Autodesk Inventor part; units mm, degrees
ref_plane "YZ Plane" through (0, 0, 0) normal (1, 0, 0) x (0, 1, 0)
ref_plane "XZ Plane" through (0, 0, 0) normal (0, 1, 0) x (-1, 0, 0)
ref_plane "XY Plane" through (0, 0, 0) normal (0, 0, 1) x (1, 0, 0)
sketch "Skizze1" plane through (0, 0, 0) normal (0, 0, 1) x (1, 0, 0)
  line L0 (-10.5, 14.5) -> (10.5, 14.5)
  line L1 (12.5, 12.5) -> (12.5, -7.362)
  line L2 (10.5, -9.362) -> (-10.5, -9.362)
  line L3 (-12.5, -7.362) -> (-12.5, 12.5)
  line L4 (-10.4, 12.5) -> (10.4, 12.5) construction
  line L5 (10.4, 12.5) -> (10.4, 0) construction
  line L6 (10.4, 0) -> (-10.4, 0) construction
  line L7 (-10.4, 0) -> (-10.4, 12.5) construction
  circle A0 centre (-10.4, 12.5) radius 1.1
  circle A1 centre (10.4, 12.5) radius 1.1
  circle A2 centre (-10.4, 0) radius 1.1
  circle A3 centre (10.4, 0) radius 1.1
  arc A4 (-10.5, 14.5) -> (-12.5, 12.5) centre (-10.5, 12.5) ccw
  arc A5 (12.5, 12.5) -> (10.5, 14.5) centre (10.5, 12.5) ccw
  arc A6 (10.5, -9.362) -> (12.5, -7.362) centre (10.5, -7.362) ccw
  arc A7 (-12.5, -7.362) -> (-10.5, -9.362) centre (-10.5, -7.362) ccw
  line L8 (0, -9.362) -> (0, 0) construction
  point P0 (-12.5, 14.5)
  point P1 (12.5, -9.362)
  point P2 (-12.5, -9.362)
  dimension "d0" = 25
  dimension "d1" = 23.862
  dimension "d2" = 2.2
  dimension "d3" = 2
  dimension "d4" = 20.8
  dimension "d5" = 12.5
  dimension "d6" = 2
extrude "Extrusion1" add sketch "Skizze1" along normal mid plane 1
sketch "Skizze2" plane through (0, 0, 0.5) normal (0, 0, 1) x (1, 0, 0)
  line L0 (-4.2, 4.2) -> (4.2, 4.2)
  line L1 (4.2, 4.2) -> (4.2, -4.2)
  line L2 (4.2, -4.2) -> (-4.2, -4.2)
  line L3 (-4.2, -4.2) -> (-4.2, 4.2)
  line L4 (-4.2, -4.2) -> (4.2, 4.2) construction
  point P0 (0, 0)
  point P1 (0, 0)
  dimension "d9" = 8.4
extrude "Extrusion2" add sketch "Skizze2" along normal blind 2.9
sketch "Skizze3" plane through (0, 0, 3.4) normal (0, 0, 1) x (1, 0, 0)
  circle A0 centre (0, 0) radius 3.6
  dimension "d12" = 7.2
extrude "Extrusion3" add sketch "Skizze3" along normal blind 1.7
sketch "Skizze4" plane through (0, 0, 5.1) normal (0, 0, 1) x (1, 0, 0)
  circle A0 centre (0, 0) radius 2.7
  circle A1 centre (0, 0) radius 0.85
  dimension "d15" = 5.4
  dimension "d16" = 1.7
extrude "Extrusion4" add sketch "Skizze4" along normal blind 0.5
sketch "Skizze5" plane through (0, 0, 0.5) normal (0, 0, 1) x (1, 0, 0)
  point P0 (0, 0)
sketch "Skizze6" plane through (0, 0, 0.5) normal (0, 0, 1) x (1, 0, 0)
  line L0 (4.2, 4.2) -> (-4.2, 4.2)
  line L1 (-3.5, 4.2) -> (3.5, 4.2)
  line L2 (3.5, 4.2) -> (3.5, 12.2)
  line L3 (3.5, 12.2) -> (-2.9111, 12.2)
  line L4 (-2.9111, 12.2) -> (-5.5, 12.2)
  line L5 (-5.5, 12.2) -> (-5.5, 8.2)
  line L6 (-5.5, 8.2) -> (-3.5, 8.2)
  line L7 (-3.5, 8.2) -> (-3.5, 4.2)
  point P0 (0, 0)
  point P1 (0, 4.2)
  dimension "d19" = 9
  dimension "d20" = 7
  dimension "d21" = 4
  dimension "d22" = 8
extrude "Extrusion5" add sketch "Skizze6" along normal blind 1.2
sketch "Skizze7" plane through (0, 0, -0.5) normal (0, 0, -1) x (-1, 0, 0)
  line L0 (-10.5, -9.362) -> (10.5, -9.362)
  line L1 (10.5, -9.362) -> (-10.5, -9.362)
  line L2 (10.4, -9.362) -> (-10.4, -9.362)
  line L3 (-10.4, -9.362) -> (-10.4, -8.212)
  line L4 (-10.4, -8.212) -> (10.4, -8.212)
  line L5 (10.4, -8.212) -> (10.4, -9.362)
  line L6 (9.75, -8.212) -> (-9.75, -8.212)
  line L7 (-9.75, -8.212) -> (-9.75, -3.762)
  line L8 (-9.75, -3.762) -> (9.75, -3.762)
  line L9 (9.75, -3.762) -> (9.75, -8.212)
  point P0 (0, 0)
  point P1 (0, -9.362)
  point P2 (0, -8.212)
  dimension "d25" = 20.8
  dimension "d26" = 1.15
  dimension "d27" = 19.5
  dimension "d28" = 5.6
extrude "Extrusion6" add sketch "Skizze7" along normal blind 2.75
sketch "Skizze8" plane through (-10.5, -9.362, 0.5) normal (0, -1, 0) x (1, 0, 0)
  line L0 (21, 0) -> (21, -1)
  line L1 (0, 0) -> (21, 0)
  line L2 (0, 0) -> (0, -1)
  line L3 (0.1, -1) -> (0, -1)
  line L4 (0.1, -1) -> (0.1, -3.75)
  line L5 (20.9, -3.75) -> (0.1, -3.75)
  line L6 (20.9, -1) -> (20.9, -3.75)
  line L7 (21, -1) -> (20.9, -1)
  line L8 (2.5, -2.18) -> (18.5, -2.18)
  line L9 (18.5, -2.18) -> (18.5, -2.55)
  line L10 (18.5, -2.55) -> (2.5, -2.55)
  line L11 (2.5, -2.55) -> (2.5, -2.18)
  line L12 (0.75, -3.75) -> (20.25, -3.75) construction
  line L13 (10.5, -3.75) -> (10.5, -2.55) construction
  line L14 (20.9, -3.75) -> (0.1, -3.75) construction
  point P0 (10.5, -0.5)
  dimension "d31" = 1.2
  dimension "d32" = 0.37
  dimension "d33" = 16
extrude "Extrusion7" cut sketch "Skizze8" against normal blind 3.5 contours L8 L9 L10 L11
ref_plane "SMD component height" through (0, 0, -1.7) normal (0, 0, -1) x (-1, 0, 0)
sketch "Skizze10" plane through (0, 0, -0.5) normal (0, 0, -1) x (-1, 0, 0)
  line L0 (12.5079, -9.362) -> (-12.5079, -9.362) construction
  line L1 (-12.5079, -9.362) -> (-12.5079, 14.5) construction
  line L2 (-12.5079, 14.5) -> (12.5079, 14.5) construction
  line L3 (12.5079, 14.5) -> (12.5079, -9.362) construction
  line L4 (10.5, 14.5) -> (-10.5, 14.5)
  line L5 (-10.4, -9.362) -> (10.4, -9.362)
  point P0 (0, 0)
  point P1 (0, 14.5)
  point P2 (0, -9.362)
decal "Aufkleber1"
sketch "Skizze11" plane through (0, 0, -3.25) normal (0, 0, -1) x (-1, 0, 0)
  line L0 (10.5, 14.5) -> (-10.5, 14.5)
  line L1 (12.5079, -9.362) -> (-12.5079, -9.362) construction
  line L2 (-12.5079, -9.362) -> (-12.5079, 14.5) construction
  line L3 (-12.5079, 14.5) -> (12.5079, 14.5) construction
  line L4 (12.5079, 14.5) -> (12.5079, -9.362) construction
  line L5 (-10.4, -9.362) -> (10.4, -9.362)
  point P0 (0, 0)
  point P1 (0, -9.362)
  point P2 (0, 14.5)
decal "Aufkleber2"
sketch "Skizze12" plane through (-10.5, -9.362, 0.5) normal (0, -1, 0) x (1, 0, 0)
  line L0 (20.9, -1) -> (20.9, -3.75)
  line L1 (0.1, -1) -> (0.1, -3.75)
  line L2 (20.9, -1) -> (0.1, -1)
  line L3 (0.1, -1) -> (0.1, -1.01)
  line L4 (0.1, -1.01) -> (20.9, -1.01)
  line L5 (20.9, -1.01) -> (20.9, -1)
  point P0 (10.5, -0.5)
  dimension "d58" = 0.01
extrude "Extrusion9" cut sketch "Skizze12" against normal blind 0.01
properties part number "Raspberry Camera V2.1"
Model file for the job. Use its own axes, mm. A direction names the side the tool comes from. Give positions to 0.01 mm unless a question says otherwise; leave off trailing zeros. Loops run counter-clockwise (first coordinate to the right, second up) from the corner with the lowest first, then second, coordinate; pieces in that order, holes last. Notation, with made-up numbers: (71, 68) - (77, 68) arc R33 cw to (77, 100) - close; hole circle Ø3 at (31, 37). An arc over 180 degrees is marked (long way). One line per item, written item: value. Start each with the question number.
1. Slice it at C-C (z = 2.5). List the corners of the cut face in (x, y), plus the area to 3 significant figures.
2. Probe L1, parallel to Y at x = -10.4, z = 0.2; L2, parallel to Y at x = 0, z = 5.2; L3, parallel to Z at x = 3.25, y = -7.75. List the from-to ranges inside material, lowest first. Write a range as from..to.
3. Which spindle directions (+Z, -Z, +X, -X, +Y, -Y) get a long thin tool onto all of the face, cutting with end or side? Do faces 4 (the flat face through (0, -8, -1.68)), 5 (the flat face through (10.4, -9, -2)), 6 (the flat face through (3.5, 8, 1)), 7 (the flat face through (-5, 8.2, 1)), 8 (the flat face through (-4.2, 0, 2)). Say none if no direction does.
4. Pin check, flat tips, straight feed: pin 1 (1 mm diameter, centred on x = -8, y = -3, fed in from -Z); pin 2 (2 mm diameter, centred on y = -5.5, z = -2.5, fed in from +X); pin 3 (10 mm diameter, centred on x = 7.5, y = 8, fed in from +Z); pin 4 (1.3 mm diameter, centred on x = 10.4, y = 12.5, fed in from -Z) (3 decimals). Stop position of each tip, or through.
5. Slice it at A-A (y = 0). List the corners of the cut face in (x, z), plus the area to 4 significant figures.
6. Pull direction X, two halves, no side cores. Call faces 1 (the cylindrical face through (-0.18, 0.83, 5.35)), 2 (the flat face through (4.2, 0, 2)), 3 (the flat face through (0, -7, -3.25)): pulls with the +X half, pulls with the -X half, needs draft (parallel to the pull), parting line crosses it, or undercut.
Solution:
1. outline: (-4.2, -4.2) - (4.2, -4.2) - (4.2, 4.2) - (-4.2, 4.2) - close
1. area: 70.6 mm^2
2. L1: y = -9.36..-1.1, 1.1..11.4, 13.6..14.5
2. L2: y = -2.7..-0.85, 0.85..2.7
2. L3: z = -3.25..-2.05, -1.68..0.5
3. face 4: -Y
3. face 5: -Z, +X, +Y, -Y
3. face 6: +Z, +X, +Y
3. face 7: +Z, -X
3. face 8: +Z, -X, -Y
4. pin 1: stops at z = -0.5
4. pin 2: stops at x = 9.75
4. pin 3: stops at z = 1.7
4. pin 4: passes through
5. outline: (-12.5, -0.5) - (-11.5, -0.5) - (-11.5, 0.5) - (-12.5, 0.5) - close; (-9.3, -0.5) - (9.3, -0.5) - (9.3, 0.5) - (4.2, 0.5) - (4.2, 3.4) - (3.6, 3.4) - (3.6, 5.1) - (2.7, 5.1) - (2.7, 5.6) - (0.85, 5.6) - (0.85, 5.1) - (-0.85, 5.1) - (-0.85, 5.6) - (-2.7, 5.6) - (-2.7, 5.1) - (-3.6, 5.1) - (-3.6, 3.4) - (-4.2, 3.4) - (-4.2, 0.5) - (-9.3, 0.5) - close; (11.5, -0.5) - (12.5, -0.5) - (12.5, 0.5) - (11.5, 0.5) - close
5. area: 59.05 mm^2
6. face 1: undercut
6. face 2: pulls with the +X half
6. face 3: needs draft
